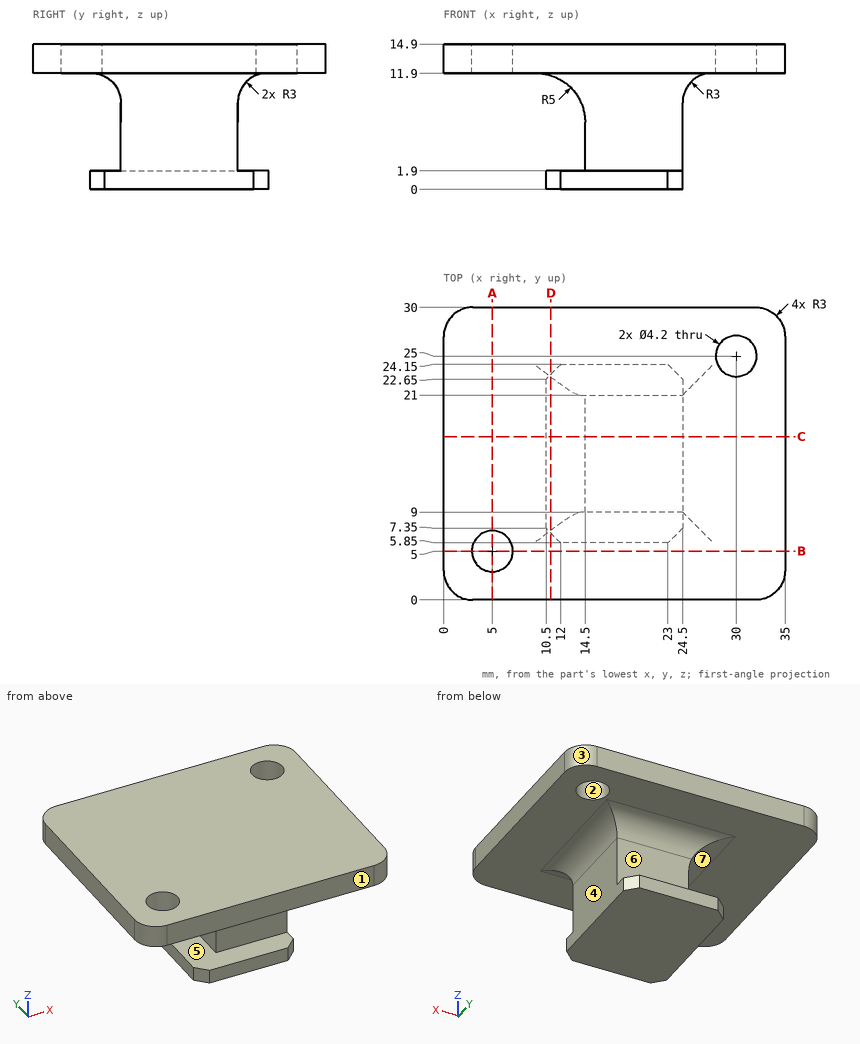
Geometry: see drawing. Coordinates: mm, zero at the bounding-box minimum. A direction names the side the tool comes from. Coordinates: 2 decimals unless noted, no trailing zeros. Order: outer loops, then holes, each group sorted by start corner. A loop starts at its lowest first (then second) coordinate and runs counter-clockwise, first axis right, second up. Notation, with made-up numbers: (-3.75, 16.5) - (41.25, 16.5) arc R18 ccw to (41.25, 38.5) - close; hole circle Ø9 at (66.25, -20.5). An arc over 180 degrees is marked (long way). Use one line per item in the form item = value.
1) Pin query (flat end, axial travel): pin 1 (2.5 mm diameter, centred on y = 12.5, z = 4, fed in from +X); pin 2 (5 mm diameter, centred on x = 14, z = 6, fed in from -Y); pin 3 (1 mm diameter, centred on x = 16.5, z = 1.5, fed in from -Y); pin 4 (1.5 mm diameter, centred on x = 3.5, z = 10, fed in from +Y). Return the tip coordinate at first contact, or that it passes through.
Solutions:
pin_1 = 24.5
pin_2 = 9
pin_3 = 5.85
pin_4 = through
2) Section C-C (y = 16.75). Return loops of the section in (x, z).
Solutions:
outline = (0, 11.9) - (9.5, 11.9) arc R5 cw to (14.5, 6.9) - (14.5, 1.9) - (10.5, 1.9) - (10.5, 0) - (24.5, 0) - (24.5, 8.9) arc R3 cw to (27.5, 11.9) - (35, 11.9) - (35, 14.9) - (0, 14.9) - close
3) Section B-B (y = 5). Return loops of the section in (x, z).
Solutions:
outline = (0, 11.9) - (2.9, 11.9) - (2.9, 14.9) - (0, 14.9) - close; (7.1, 11.9) - (35, 11.9) - (35, 14.9) - (7.1, 14.9) - close
4) Mould query, pull axis X, two halves, no side actions, for the marked faces 1, 2 and 3. Classes: +X half, -X half, draft (parallel to the pull), parting line (faces both ways), or undercut.
Solutions:
face_1 = draft
face_2 = undercut
face_3 = +X half
5) Section D-D (x = 11). Return loops of the section in (y, z), then the cut area to 3 significant figures.
Solutions:
outline = (0, 11.9) - (6, 11.9) arc R3 cw to (7.15, 11.67) - (22.85, 11.67) arc R3 cw to (24, 11.9) - (30, 11.9) - (30, 14.9) - (0, 14.9) - close; (6.85, 0) - (23.15, 0) - (23.15, 1.9) - (6.85, 1.9) - close
area = 125 mm^2
6) Set-up query: the marked faces 4, 5, 6 and 7. Return all of +Z, -Z, +X, -X, +Y, -Y with unobstructed straight access to the full face (end or side cutting, diameter ignored); none if empty.
Solutions:
face_4 = -Z, +X, +Y, -Y
face_5 = -X
face_6 = +X, -X, +Y
face_7 = -X, +Y, -Y
7) Section A-A (x = 5). Return loops of the section in (y, z), then the cut area to 3 significant figures.
Solutions:
outline = (0, 11.9) - (2.9, 11.9) - (2.9, 14.9) - (0, 14.9) - close; (7.1, 11.9) - (30, 11.9) - (30, 14.9) - (7.1, 14.9) - close
area = 77.4 mm^2
8) Ray query, L1, parallel to X at y = 5, z = 12.7; L2, parallel to Y at x = 30, z = 12.8; L3, parallel to Y at x = 5, z = 13.9. Return the intervals inside material, ascending.
Solutions:
L1 = 0 to 2.9, 7.1 to 35
L2 = 0 to 22.9, 27.1 to 30
L3 = 0 to 2.9, 7.1 to 30
